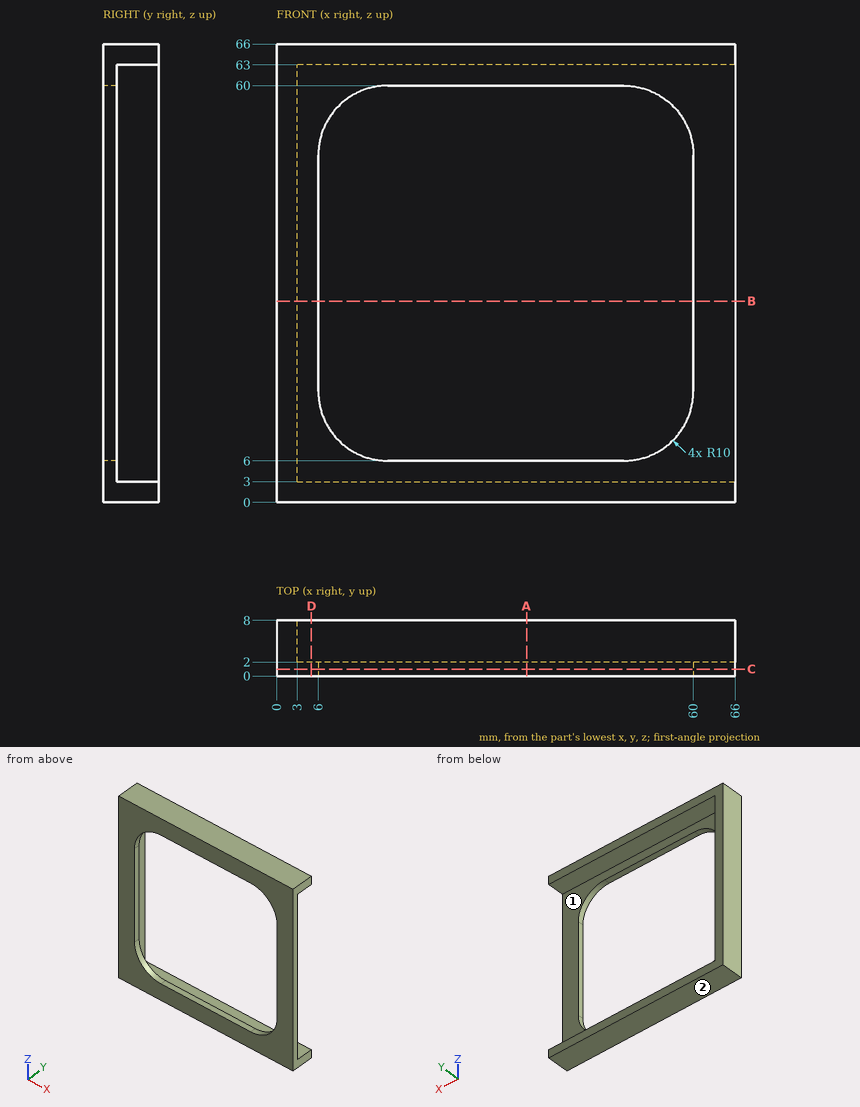
Check sheet for the drawn part. Datum: minimum x, y, z corner. Units: mm. A direction names the side the tool comes from. Round coordinates to 2 decimals unless told otherwise and drop trailing zeros. Order: outer loops, then holes, each group sorted by start corner. A loop starts at its lowest first (then second) coordinate and runs counter-clockwise, first axis right, second up.
(1) Access from +Z, -Z, +X, -X, +Y, -Y to the whole of each face (thin tool, end or side, straight path). Record for the marked faces 1 and 2.
(2) Cross-section at A-A, the plane x = 36. Enter the section's corners in (y, z).
(3) Cross-section at D-D, the plane x = 5. Enter the section's corners in (y, z), and give its area (3 significant figures).
(4) Scan lines: probe 1 along Z at (x, y) = (43.5, 3.5); probe 2 along Z at (x, y) = (48.5, 1). Record each from-to range of solid material in increasing order.
(5) Cross-section at C-C, the plane y = 1. Enter the section's corners in (x, z), and give its area (3 significant figures).
(6) Cross-section at B-B, the plane z = 29. Enter the section's corners in (x, y).
(7) Go/stop test with a flat-tipped pin: P1, Ø3, axis at y = 6, z = 30, coming from the +X side. Record where the tip stops, or that it passes through.
Check sheet entries:
1. face 1: +X, +Y
1. face 2: -Z, +X, -X, +Y, -Y
2. outline: (0, 0) - (8, 0) - (8, 3) - (2, 3) - (2, 6) - (0, 6) - close; (0, 60) - (2, 60) - (2, 63) - (8, 63) - (8, 66) - (0, 66) - close
3. outline: (0, 0) - (8, 0) - (8, 3) - (2, 3) - (2, 63) - (8, 63) - (8, 66) - (0, 66) - close
3. area: 168 mm2
4. probe 1: z = 0 to 3, 63 to 66
4. probe 2: z = 0 to 6, 60 to 66
5. outline: (0, 0) - (66, 0) - (66, 66) - (0, 66) - close; hole (6, 16) arc R10 ccw to (16, 6) - (50, 6) arc R10 ccw to (60, 16) - (60, 50) arc R10 ccw to (50, 60) - (16, 60) arc R10 ccw to (6, 50) - close
5. area: 1,530 mm2
6. outline: (0, 0) - (6, 0) - (6, 2) - (3, 2) - (3, 8) - (0, 8) - close; (60, 0) - (66, 0) - (66, 2) - (60, 2) - close
7. P1: stops at x = 3
